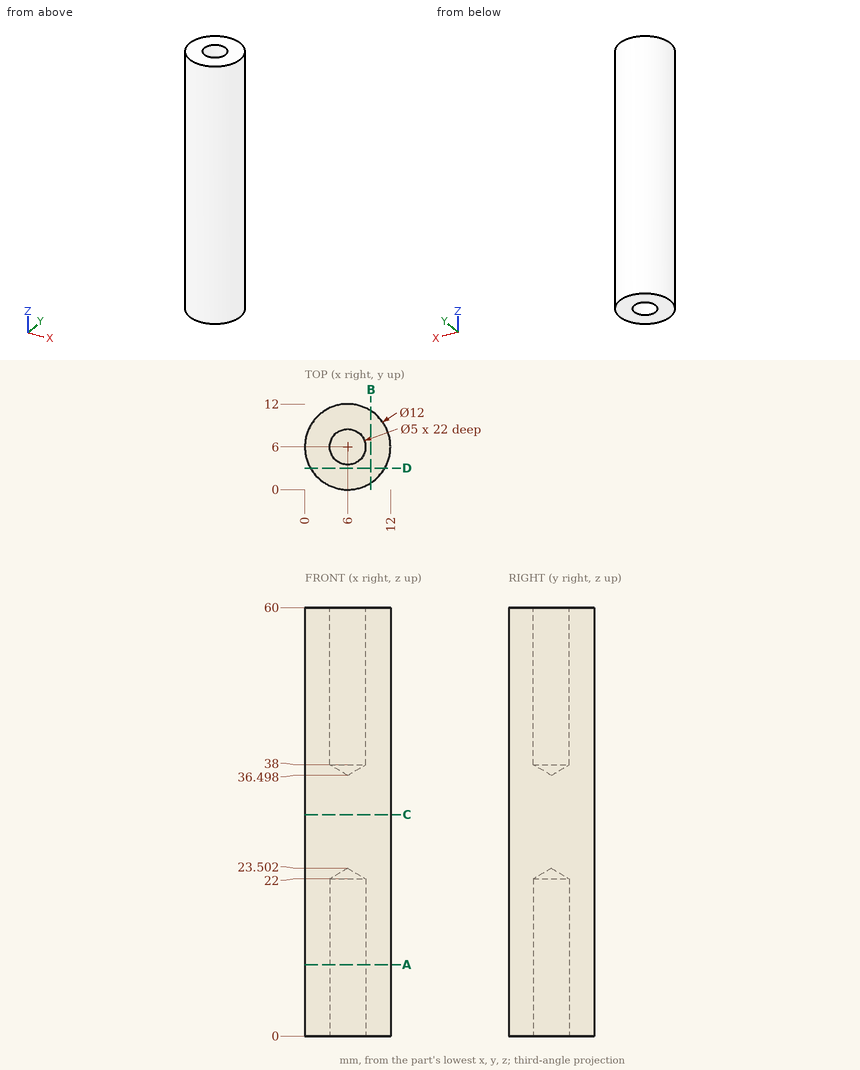
Answer from the drawing. Dimensions are ordinates in mm from the lowest x, y and z of the part. Give positions to 0.01 mm unless a question says otherwise; leave off trailing zeros. Loops run counter-clockwise (first coordinate to the right, second up) from the corner with the lowest first, then second, coordinate; pieces in that order, holes last. Notation, with made-up numbers: (-36, 45) -> (-15, 45) arc R29 cw to (-15, 78) -> close; hole circle Ø11 at (42.5, 72.25). An arc over 180 degrees is marked (long way). One line per question, with ' | ' between items. Start each with the question number.
1) Straight lines are drawn through the part: L1, parallel to Y at x = 6, z = 7.5; L2, parallel to X at y = 4.75, z = 39 (1 decimal); L3, parallel to X at y = 4, z = 40. For each, find the intervals that lie inside material, in ascending order.
2) Section D-D, the plane y = 3 is taken. Determine the outline of the cut face in (x, z).
3) Section C-C, the plane z = 31 is taken. Determine the outline of the cut face in (x, y).
4) Section B-B, the plane x = 9.25 is taken. Determine the outline of the cut face in (y, z), then the cut area to 3 significant figures.
5) Each of these flat-tipped pins is pushed along its axis until it touches: pin 1 (1 mm diameter, centred on x = 8.5, y = 10, fed in from -Z); pin 2 (1 mm diameter, centred on x = 8, z = 25, fed in from +Y); pin 3 (1 mm diameter, centred on y = 10.5, z = 49.5, fed in from +X); pin 4 (1.5 mm diameter, centred on y = 5, z = 26.5, fed in from -X). Where does it stop, or does it pass through?
6) Section A-A, the plane z = 10 is taken. Determine the outline of the cut face in (x, y).
Resolved:
1) L1: 0 to 3.5, 8.5 to 12 | L2: 0.1 to 3.8, 8.2 to 11.9 | L3: 0.34 to 4.5, 7.5 to 11.66
2) outline: (0.8, 0) -> (11.2, 0) -> (11.2, 60) -> (0.8, 60) -> close
3) outline: circle Ø12 at (6, 6)
4) outline: (0.96, 0) -> (11.04, 0) -> (11.04, 60) -> (0.96, 60) -> close | area: 605 mm2
5) pin 1: z = 0 | pin 2: y = 11.81 | pin 3: x = 10.47 | pin 4: x = 0.01
6) outline: circle Ø12 at (6, 6); hole circle Ø5 at (6, 6)
